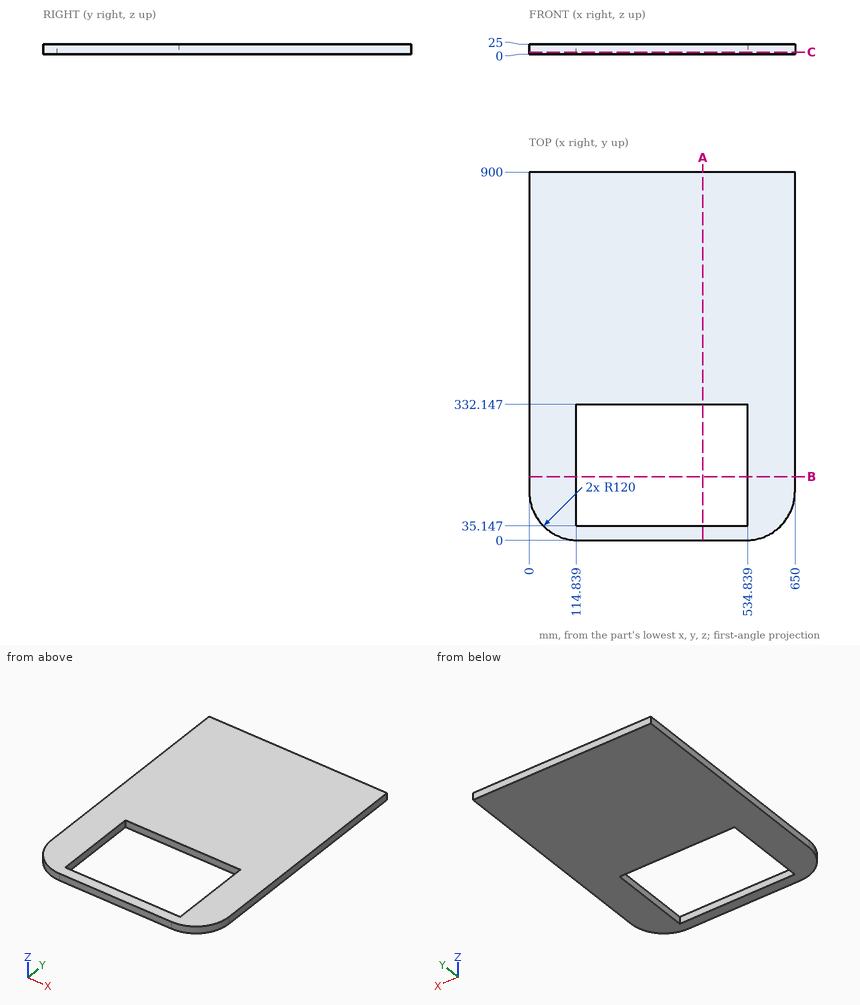
Print and shaded views of the part. All mm, measured from the part's lowest x, y and z. Coordinates: 2 decimals unless noted, no trailing zeros. Loops run counter-clockwise (first coordinate to the right, second up) from the corner with the lowest first, then second, coordinate; pieces in that order, holes last. Notation, with made-up numbers: M 40,-0.5 L 80,-0.5 A6 cw 80,10.5 Z; hole C 11.5,69 d2. An arc over 180 degrees is marked long. Use a Markdown table: item, result. Add a question column.
Q1. Cut at B-B (y = 155.5). Write the cut outline in (x, z), and give its area (3 significant figures).
Q2. Probe L1, parallel to Y at x = 319, z = 24; L2, parallel to X at y = 190, z = 20; L3, parallel to Y at x = 116.5, z = 13. List the from-to ranges inside material, lowest first.
Q3. Pin check, flat tip, straight feed: P1, Ø7.5, axis at y = 111.5, z = 18, coming from the -X side. Stop position of the tip, or through.
Q4. Cut at C-C (z = 5). Write the cut outline in (x, y), and give its area (3 significant figures).
Q5. Cut at A-A (x = 425). Write the cut outline in (y, z).
Worked out:
| question | item | result |
|---|---|---|
| 1 | outline | M 0,0 L 114.84,0 L 114.84,25 L 0,25 Z; M 534.84,0 L 650,0 L 650,25 L 534.84,25 Z |
| 1 | area | 5,750 mm2 |
| 2 | L1 | y = 0 to 35.15, 332.15 to 900 |
| 2 | L2 | x = 0 to 114.84, 534.84 to 650 |
| 2 | L3 | y = 0.05 to 35.15, 332.15 to 900 |
| 3 | P1 | stops at x = 0.09 |
| 4 | outline | M 0,120 A120 ccw 120,0 L 530,0 A120 ccw 650,120 L 650,900 L 0,900 Z; hole M 114.84,35.15 L 534.84,35.15 L 534.84,332.15 L 114.84,332.15 Z |
| 4 | area | 454,000 mm2 |
| 5 | outline | M 0,0 L 35.15,0 L 35.15,25 L 0,25 Z; M 332.15,0 L 900,0 L 900,25 L 332.15,25 Z |
